Autodesk Inventor part; units mm, degrees
ref_plane "YZ Plane" through (0, 0, 0) normal (1, 0, 0) x (0, 1, 0)
ref_plane "XZ Plane" through (0, 0, 0) normal (0, 1, 0) x (-1, 0, 0)
ref_plane "XY Plane" through (0, 0, 0) normal (0, 0, 1) x (1, 0, 0)
sketch "Sketch1" plane through (0, 0, 0) normal (0, 0, 1) x (1, 0, 0)
  line L0 (-51.7767, -125) -> (-125, -51.7767)
  line L1 (-125, -51.7767) -> (-125, 51.7767)
  line L2 (-125, 51.7767) -> (-51.7767, 125)
  line L3 (-51.7767, 125) -> (51.7767, 125)
  line L4 (51.7767, 125) -> (125, 51.7767)
  line L5 (125, 51.7767) -> (125, -51.7767)
  line L6 (125, -51.7767) -> (51.7767, -125)
  line L7 (51.7767, -125) -> (-51.7767, -125)
  circle A0 centre (11.5, -120) radius 1.5
  circle A1 centre (-11.5, -120) radius 1.5
  circle A2 centre (120, 11.5) radius 1.5
  circle A3 centre (120, -11.5) radius 1.5
  circle A4 centre (-11.5, 120) radius 1.5
  circle A5 centre (11.5, 120) radius 1.5
  circle A6 centre (-120, -11.5) radius 1.5
  circle A7 centre (-120, 11.5) radius 1.5
  point P0 (0, 0)
  point P1 (0, 0)
  dimension "d0" = 250
  dimension "d1" = 3
  dimension "d2" = 3
  dimension "d3" = 5
  dimension "d4" = 5
  dimension "d5" = 11.5
  dimension "d6" = 11.5
  dimension "d9" = 360
extrude "Extrusion1" add sketch "Sketch1" along normal blind 8
sketch "dm" plane through (0, 0, 8) normal (0, 0, 1) x (1, 0, 0)
  line L0 (-37.5, 37.5) -> (37.5, 37.5) construction
  line L1 (37.5, 37.5) -> (37.5, -37.5) construction
  line L2 (37.5, -37.5) -> (-37.5, -37.5) construction
  line L3 (-37.5, -37.5) -> (-37.5, 37.5) construction
  line L4 (-125.8266, 126.5) -> (127.1734, 126.5)
  line L5 (127.1734, 126.5) -> (127.1734, -126.5)
  line L6 (127.1734, -126.5) -> (-125.8266, -126.5)
  line L7 (-125.8266, -126.5) -> (-125.8266, 126.5)
  line L8 (-125.8266, 126.5) -> (127.1734, -126.5) construction
  line L9 (127.1734, 126.5) -> (-125.8266, -126.5) construction
  point P0 (0, 0)
  point P1 (0.6734, 0)
  dimension "d14" = 75
  dimension "d31" = 253
  dimension "d32" = 253
  dimension "d35" = 37.5
  dimension "d36" = 37.5
  dimension "d44" = 37.5
decal "Decal1"
sketch "Sketch3" plane through (0, 0, 8) normal (0, 0, 1) x (1, 0, 0)
  line L0 (51.7767, -125) -> (125, -51.7767)
  line L1 (125, -51.7767) -> (125, 51.7767)
  line L2 (125, 51.7767) -> (51.7767, 125)
  line L3 (51.7767, 125) -> (-51.7767, 125)
  line L4 (-51.7767, 125) -> (-125, 51.7767)
  line L5 (-125, 51.7767) -> (-125, -51.7767)
  line L6 (-125, -51.7767) -> (-51.7767, -125)
  line L7 (-51.7767, -125) -> (51.7767, -125)
  circle A0 centre (-120, 11.5) radius 1.5
  circle A1 centre (-120, -11.5) radius 1.5
  circle A2 centre (11.5, 120) radius 1.5
  circle A3 centre (-11.5, 120) radius 1.5
  circle A4 centre (120, -11.5) radius 1.5
  circle A5 centre (120, 11.5) radius 1.5
  circle A6 centre (-11.5, -120) radius 1.5
  circle A7 centre (11.5, -120) radius 1.5
  point P0 (0, 0)
equation "\"d4\" = d3"
properties part number "Plate_Acrylic" material "Polycarbonate, Clear"
The model under review builds one solid part; all positions refer to its coordinate system, in mm. Give positions to 0.01 mm unless a question says otherwise; leave off trailing zeros. Write each loop counter-clockwise with the first axis right and the second up, starting at its lowest first coordinate (ties: lowest second). Pieces come first, ordered by that corner, then holes. Notation, with made-up numbers: (51.25, -18) - (102.25, -18) arc R14 ccw to (102.25, -2) - close; hole circle Ø5 at (60, -33). An arc over 180 degrees is marked (long way). Answer in a Markdown table with one row per item. Add a question column.
1. We need section A-A on z = 4.5. State how many separate pieces and enclosed holes the cut face has, then the cut area to 3 significant figures.
2. Insertion check: P1, Ø4, axis at x = 70.5, z = 5.5, coming from the -Y side; P2, Ø2.5, axis at x = -11.5, y = 120, coming from the +Z side. Each pin has a flat end and moves straight along its axis. Give the tip position at first contact, or say it passes through.
3. We need section C-C on y = 98.5. Write out the cut boundary in (x, z).
4. Wall thickness on line 1 along Y through (x, z) = (-11.5, 3); line 2 along Y through (x, z) = (-120, 6): over which ranges is each line inside the solid? List them lowest first. Write a range as [from, to].
5. We need section B-B on x = -92. Write out the cut boundary in (y, z).
Ans:
| question | item | result |
|---|---|---|
| 1 | separate pieces | 1 |
| 1 | enclosed holes | 8 |
| 1 | area | 51,700 mm^2 |
| 2 | P1 | stops at y = -108.28 |
| 2 | P2 | passes through |
| 3 | outline | (-78.28, 0) - (78.28, 0) - (78.28, 8) - (-78.28, 8) - close |
| 4 | line 1 | y = [-125, -121.5], [-118.5, 118.5], [121.5, 125] |
| 4 | line 2 | y = [-56.78, -13], [-10, 10], [13, 56.78] |
| 5 | outline | (-84.78, 0) - (84.78, 0) - (84.78, 8) - (-84.78, 8) - close |
